from build123d import *

# Parameters (mm, degrees)
BOSS_EXTRUDE3_DEPTH   = 3.175
F_3_0MM_DOWEL_HOLE1_D = 3


with BuildPart() as part:
    # Sketch7 → Boss-Extrude3 (new, symmetric)
    with BuildSketch(Plane(origin=(0, 0, 0), x_dir=(1, 0, 0), z_dir=(0, 1, 0))):
        Polygon((-12.7, -32.5), (-12.7, -40), (12.7, -40), (12.7, -32.5), (6.7564, -32.5), (6.7564, 32.5), (12.7, 32.5), (12.7, 40), (-12.7, 40), (-12.7, 32.5), (-6.7564, 32.5), (-6.7564, -32.5), align=None)
    extrude(amount=BOSS_EXTRUDE3_DEPTH, both=True)

    # Ø3.0mm Dowel Hole1 (through all)
    with Locations(Plane(origin=(0, 0, -40), x_dir=(-1, 0, 0), z_dir=(0, 0, -1))):
        with Locations((-9.779, 0), (9.779, 0)):
            Hole(F_3_0MM_DOWEL_HOLE1_D / 2)


solid = part.part
The listing builds one solid part. Answer for the finished solid, in the listing's coordinates (mm). A direction names the side the tool comes from. Coordinates: 2 decimals unless noted, no trailing zeros. Write each loop counter-clockwise with the first axis right and the second up, starting at its lowest first coordinate (ties: lowest second). Pieces come first, ordered by that corner, then holes. Notation, with made-up numbers: (-32, 80) - (-26, 80) arc R29 cw to (-26, 117) - close; hole circle Ø7 at (0, -21). An arc over 180 degrees is marked (long way). Return JSON: item names as keys, results as strings.
1. The part is cut by section D-D on z = -24. Determine the outline of the cut face in (x, y) (3 decimals), then the cut area to 3 significant figures.
Final values:
{"outline": "(-6.756, -3.175) - (6.756, -3.175) - (6.756, 3.175) - (-6.756, 3.175) - close", "area": "85.8 mm^2"}
2. The part is cut by section A-A on y = 0. Determine the outline of the cut face in (x, z).
Final values:
{"outline": "(-12.7, -40) - (-11.28, -40) - (-11.28, -32.5) - (-12.7, -32.5) - close; (-12.7, 32.5) - (-11.28, 32.5) - (-11.28, 40) - (-12.7, 40) - close; (-8.28, -40) - (8.28, -40) - (8.28, -32.5) - (6.76, -32.5) - (6.76, 32.5) - (8.28, 32.5) - (8.28, 40) - (-8.28, 40) - (-8.28, 32.5) - (-6.76, 32.5) - (-6.76, -32.5) - (-8.28, -32.5) - close; (11.28, -40) - (12.7, -40) - (12.7, -32.5) - (11.28, -32.5) - close; (11.28, 32.5) - (12.7, 32.5) - (12.7, 40) - (11.28, 40) - close"}
3. For a pull along Z with two mould halves and no side action, classify faces 4 (the face through (6.756, 0, 0)), 5 (the face through (-11.278, 0.066, -36.198)), 6 (the face through (0, 0, 40)) as +Z half, -Z half, draft (parallel to the pull), parting line (faces both ways), or undercut.
Final values:
{"face 4": "undercut", "face 5": "draft", "face 6": "+Z half"}
4. The part is cut by section B-B on x = -9.75. Determine the outline of the cut face in (y, z) (3 decimals).
Final values:
{"outline": "(-3.175, -40) - (-1.5, -40) - (-1.5, -32.5) - (-3.175, -32.5) - close; (-3.175, 32.5) - (-1.5, 32.5) - (-1.5, 40) - (-3.175, 40) - close; (1.5, -40) - (3.175, -40) - (3.175, -32.5) - (1.5, -32.5) - close; (1.5, 32.5) - (3.175, 32.5) - (3.175, 40) - (1.5, 40) - close"}
5. Consider line 1 along Z through (x, y) = (9.5, -2); line 2 along X through (y, z) = (2.5, 27); line 3 along Y through (x, z) = (9.5, 33.5) (3 decimals). Determine where each line is inside the solid, lowest interval first.
Final values:
{"line 1": "-40 to -32.5, 32.5 to 40", "line 2": "-6.76 to 6.76", "line 3": "-3.175 to -1.474, 1.474 to 3.175"}
6. Which of the six approach directions +Z, -Z, +X, -X, +Y, -Y give full straight-line access (tool end or side, diameter ignored) to faces 1 (the face through (-6.756, 0, 0)), 2 (the face through (8, 1, 32.5)), 3 (the face through (12.7, 0, 36))?
Final values:
{"face 1": "-X, +Y, -Y", "face 2": "+X, +Y, -Y", "face 3": "+Z, -Z, +X, +Y, -Y"}
7. The part is cut by section C-C on z = 34. Determine the outline of the cut face in (x, y) (3 decimals), then the cut area to 3 significant figures.
Final values:
{"outline": "(-12.7, -3.175) - (12.7, -3.175) - (12.7, 3.175) - (-12.7, 3.175) - close; hole circle Ø3 at (-9.779, 0); hole circle Ø3 at (9.779, 0)", "area": "147 mm^2"}
8. Each of these flat-tipped pins is pushed along its axis until it touches: pin 1 Ø3 at (y, z) = (1.5, -3.5) entering from -X; pin 2 Ø2 at (y, z) = (2.5, -4.5) entering from +X. Where does it stop, or does it pass through?
Final values:
{"pin 1": "x = -6.76", "pin 2": "x = 6.76"}
